Check sheet for the modelled part. Datum: model origin and axes. Units: mm. A direction names the side the tool comes from. Round coordinates to 2 decimals unless told otherwise and drop trailing zeros. Write each loop counter-clockwise with the first axis right and the second up, starting at its lowest first coordinate (ties: lowest second). Pieces come first, ordered by that corner, then holes. Notation, with made-up numbers: (-39.75, 55) -> (-34.75, 55) arc R31 cw to (-34.75, 80) -> close; hole circle Ø9 at (-23, 36.5). An arc over 180 degrees is marked (long way). One line per item, written item: value.
from build123d import *

# Parameters (mm, degrees)
SKETCH1_W           = 270
SKETCH1_H           = 110
BOSS_EXTRUDE1_DEPTH = 4
BOSS_EXTRUDE2_DEPTH = 30
SKETCH3_R           = 3
CUT_EXTRUDE1_DEPTH  = 30


with BuildPart() as part:
    # Sketch1 → Boss-Extrude1 (new body)
    with BuildSketch(Plane.XY):
        Rectangle(SKETCH1_W, SKETCH1_H)
    extrude(amount=BOSS_EXTRUDE1_DEPTH)

    # Sketch2 → Boss-Extrude2 (add)
    with BuildSketch(Plane.XY.offset(4)):
        Polygon((-128.071344503, 55), (-135, 55), (-113.784719429, 40), (-113.784719429, -55), (-109.784719429, -55), (-109.784719429, 42.070669408), align=None)
        Polygon((128.071344503, 55), (109.784719429, 42.070669408), (109.784719429, -55), (113.784719429, -55), (113.784719429, 40), (135, 55), align=None)
    extrude(amount=BOSS_EXTRUDE2_DEPTH)

    # Sketch3 → Cut-Extrude1 (cut)
    with BuildSketch(Plane.XY.offset(4)):
        with Locations((-120, -46)):
            Circle(SKETCH3_R)
        with Locations((120, -46)):
            Circle(SKETCH3_R)
        with Locations((127, 46)):
            Circle(SKETCH3_R)
        with Locations((-127, 46)):
            Circle(SKETCH3_R)
    extrude(amount=-CUT_EXTRUDE1_DEPTH, mode=Mode.SUBTRACT)


solid = part.part
Item 1: Sectioned sample at B-B (z = 6.5). Enter the section's corners in (x, y), then the cut area to 3 significant figures.
Result set:
outline: (-135, 55) -> (-113.78, 40) -> (-113.78, -55) -> (-109.78, -55) -> (-109.78, 42.07) -> (-128.07, 55) -> close; (109.78, -55) -> (113.78, -55) -> (113.78, 40) -> (135, 55) -> (128.07, 55) -> (109.78, 42.07) -> close
area: 962 mm^2
Item 2: Sectioned sample at D-D (x = -120). Enter the section's corners in (y, z).
Result set:
outline: (-55, 0) -> (-49, 0) -> (-49, 4) -> (-55, 4) -> close; (-43, 0) -> (55, 0) -> (55, 4) -> (49.29, 4) -> (49.29, 34) -> (44.39, 34) -> (44.39, 4) -> (-43, 4) -> close
Item 3: Depth check by flat-ended pin: pin 1 (5 mm diameter, centred on x = 16, y = -16.5, fed in from +Z); pin 2 (15 mm diameter, centred on y = -3.5, z = 19, fed in from -X); pin 3 (0.7 mm diameter, centred on x = 125.5, y = 48, fed in from -Z); pin 4 (5 mm diameter, centred on x = -127, y = 46, fed in from -Z). Enter the tip coordinate at first touch or a pass-through.
Result set:
pin 1: z = 4
pin 2: x = -113.78
pin 3: z = 4
pin 4: through
Item 4: Release check for a two-part mould opening along X. For faces 1 (the cylindrical face through (-117.14, -45.1, 2.03)), 2 (the flat face through (-113.785, -7, 19)), 3 (the flat face through (124, 1, 4)) record: pulls with the +X half, pulls with the -X half, needs draft (parallel to the pull), parting line crosses it, or undercut.
Result set:
face 1: undercut
face 2: pulls with the -X half
face 3: needs draft
Item 5: Material ranges on line 1 along X through (y, z) = (46, 2); line 2 along Y through (x, z) = (-120, 1); line 3 along Y through (x, z) = (127, 1.1), recorded low to high.
Result set:
line 1: -135 to -130, -124 to 124, 130 to 135
line 2: -55 to -49, -43 to 55
line 3: -55 to 43, 49 to 55
Item 6: Sectioned sample at A-A (y = -46). Enter the section's corners in (x, z), then the cut area to 3 significant figures.
Result set:
outline: (-135, 0) -> (-123, 0) -> (-123, 4) -> (-135, 4) -> close; (-117, 0) -> (117, 0) -> (117, 4) -> (113.78, 4) -> (113.78, 34) -> (109.78, 34) -> (109.78, 4) -> (-109.78, 4) -> (-109.78, 34) -> (-113.78, 34) -> (-113.78, 4) -> (-117, 4) -> close; (123, 0) -> (135, 0) -> (135, 4) -> (123, 4) -> close
area: 1,270 mm^2
Item 7: Tool access check on faces 4 (the flat face through (119.06, 48.63, 18.79)), 5 (the flat face through (-124.541, 47.605, 18.79)), 6 (the flat face through (-109.785, -7, 19)), 7 (the flat face through (124.244, 47.395, 18.79)). Record the directions out of +Z, -Z, +X, -X, +Y, -Y that give a thin tool (end or side, any length) a straight path to the whole face; none if there is none.
Result set:
face 4: +Z, +Y
face 5: +Z, -X, -Y
face 6: +Z, +Y, -Y
face 7: +Z, +X, -Y
Item 8: Sectioned sample at C-C (y = -29.5). Enter the section's corners in (x, z), then the cut area to 3 significant figures.
Result set:
outline: (-135, 0) -> (135, 0) -> (135, 4) -> (113.78, 4) -> (113.78, 34) -> (109.78, 34) -> (109.78, 4) -> (-109.78, 4) -> (-109.78, 34) -> (-113.78, 34) -> (-113.78, 4) -> (-135, 4) -> close
area: 1,320 mm^2
